Geometry check sheet. Reference: the model listing, model coordinates, mm. A direction names the side the tool comes from. Round coordinates to 2 decimals unless told otherwise and drop trailing zeros. Loops run counter-clockwise (first coordinate to the right, second up) from the corner with the lowest first, then second, coordinate; pieces in that order, holes last. Notation, with made-up numbers: (-28.75, 31.25) - (-20.75, 31.25) arc R12 cw to (-20.75, 54.25) - close; hole circle Ø10 at (28.5, 30). An arc over 180 degrees is marked (long way). Answer as CSV lines item,"result". Start each with the question number.
1) Cross-section at A-A on y = -8.5. Record the boundary of the cut face in (x, z), and give its area (3 significant figures).
2) Draft check along X on faces 1 (the flat face through (-9, 16, 2)), 2 (the cylindrical face through (18.1, 24.4, 2)), 3 (the flat face through (-14, 25.596, 2)), 4 (the cylindrical face through (-8.699, -2.965, 2.028)). Enter one of: released by +X, released by -X, zero draft, split by the parting line, or undercut.
3) Access from +Z, -Z, +X, -X, +Y, -Y to the whole of each face (thin tool, end or side, straight path). Record for faces 5 (the cylindrical face through (12.743, 5.831, 1.972)), 6 (the cylindrical face through (10.203, 24.455, 2.028)), 7 (the flat face through (0, -24.404, 2)).
4) Depth check by flat-ended pin: P1, Ø1.2, axis at x = -2.5, z = 2, coming from the +Y side. Enter the tip coordinate at first touch or a pass-through.
5) Thickness scan on line 1 along X through (y, z) = (20.5, 3.25); line 2 along X through (y, z) = (6, 3); line 3 along X through (y, z) = (-2, 3.6). Record the ranges inside material, lowest first.
6) Cross-section at C-C on z = 2. Record the boundary of the cut face in (x, y) (3 decimals), and give its area (3 significant figures).
7) Cross-section at D-D on y = 3. Record the boundary of the cut face in (x, z), and give its area (3 significant figures).
8) Cross-section at B-B on y = 17. Record the boundary of the cut face in (x, z).
from build123d import *

# Parameters (mm, degrees)
F0_R     = 1.875
F1_DEPTH = 4
F2_R     = 4
F3_R     = 1


with BuildPart() as f1:
    # F0 (on Top) → F1 (new body)
    with BuildSketch(Plane.XY):
        with BuildLine():
            Line((19.25, -24.404246), (19.25, 25.595754))
            Line((19.25, 25.595754), (9, 25.595754))
            Line((9, 25.595754), (9, 10.392248))
            ThreePointArc((9, 10.392248), (12.744, 5.75), (9, 1.107752))
            Line((9, 1.107752), (9, -3.25))
            Line((9, -3.25), (-9, -3.25))
            Line((-9, -3.25), (-9, 1.107752))
            ThreePointArc((-9, 1.107752), (-12.744, 5.75), (-9, 10.392248))
            Line((-9, 10.392248), (-9, 25.595754))
            Line((-9, 25.595754), (-19.25, 25.595754))
            Line((-19.25, 25.595754), (-19.25, -24.404246))
            Line((-19.25, -24.404246), (19.25, -24.404246))
        make_face()
        with Locations((-14.547877, -8.5)):
            Circle(F0_R, mode=Mode.SUBTRACT)
        with Locations((14.547877, -8.5)):
            Circle(F0_R, mode=Mode.SUBTRACT)
        with Locations((-14.547877, 20.595754)):
            Circle(F0_R, mode=Mode.SUBTRACT)
        with Locations((14.547877, 20.595754)):
            Circle(F0_R, mode=Mode.SUBTRACT)
    extrude(amount=F1_DEPTH)

    # F2
    f2_edges = [f1.edges().sort_by_distance(p)[0] for p in [
        (19.25, 25.595754, 2),
        (-19.25, 25.595754, 2),
        (-9, 25.595754, 2),
        (9, 25.595754, 2),
    ]]
    fillet(f2_edges, radius=F2_R)

    # F3
    f3_edges = [f1.edges().sort_by_distance(p)[0] for p in [
        (-9, 10.392248, 2),
        (-9, 1.107752, 2),
        (-9, -3.25, 2),
        (9, -3.25, 2),
        (9, 1.107752, 2),
        (9, 10.392248, 2),
    ]]
    fillet(f3_edges, radius=F3_R)


solid = f1.part
Answer block:
1,outline,"(-19.25, 0) - (-16.42, 0) - (-16.42, 4) - (-19.25, 4) - close; (-12.67, 0) - (12.67, 0) - (12.67, 4) - (-12.67, 4) - close; (16.42, 0) - (19.25, 0) - (19.25, 4) - (16.42, 4) - close"
1,area,"124 mm^2"
2,face 1,"undercut"
2,face 2,"released by +X"
2,face 3,"zero draft"
2,face 4,"undercut"
3,face 5,"+Z, -Z"
3,face 6,"+Z, -Z, +Y"
3,face 7,"+Z, -Z, +X, -X, -Y"
4,P1,"stops at y = -3.25"
5,line 1,"x = -19.25 to -16.42, -12.68 to -9, 9 to 12.68, 16.42 to 19.25"
5,line 2,"x = -19.25 to -12.74, 12.74 to 19.25"
5,line 3,"x = -19.25 to -9, 9 to 19.25"
6,outline,"(-19.25, -24.404) - (19.25, -24.404) - (19.25, 21.596) arc R4 ccw to (15.25, 25.596) - (13, 25.596) arc R4 ccw to (9, 21.596) - (9, 11.139) arc R1 ccw to (9.651, 10.202) arc R4.75 cw to (9.651, 1.298) arc R1 ccw to (9, 0.361) - (9, -2.25) arc R1 cw to (8, -3.25) - (-8, -3.25) arc R1 cw to (-9, -2.25) - (-9, 0.361) arc R1 ccw to (-9.651, 1.298) arc R4.75 cw to (-9.651, 10.202) arc R1 ccw to (-9, 11.139) - (-9, 21.596) arc R4 ccw to (-13, 25.596) - (-15.25, 25.596) arc R4 ccw to (-19.25, 21.596) - close; hole circle Ø3.75 at (-14.548, -8.5); hole circle Ø3.75 at (-14.548, 20.596); hole circle Ø3.75 at (14.548, -8.5); hole circle Ø3.75 at (14.548, 20.596)"
6,area,"1,300 mm^2"
7,outline,"(-19.25, 0) - (-11.87, 0) - (-11.87, 4) - (-19.25, 4) - close; (11.87, 0) - (19.25, 0) - (19.25, 4) - (11.87, 4) - close"
7,area,"59.1 mm^2"
8,outline,"(-19.25, 0) - (-9, 0) - (-9, 4) - (-19.25, 4) - close; (9, 0) - (19.25, 0) - (19.25, 4) - (9, 4) - close"
